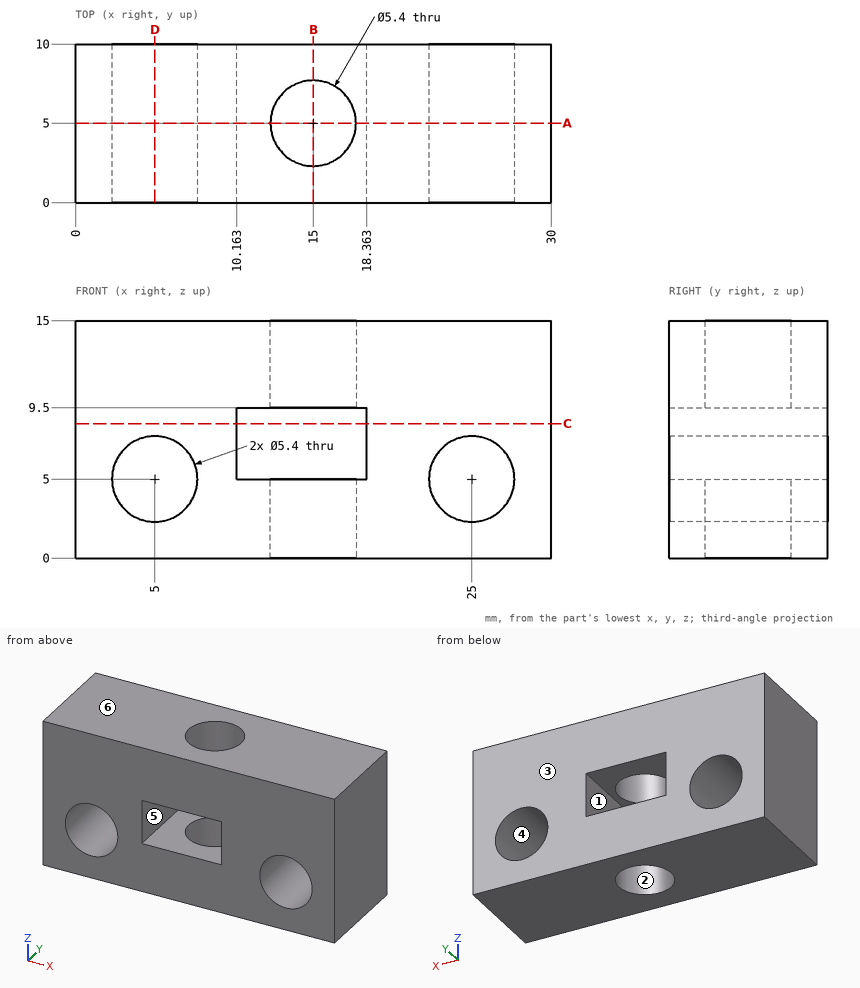
Geometry check sheet. Reference: drawing and pictorial views, mm from the part's lowest x, y, z. A direction names the side the tool comes from. Give positions to 0.01 mm unless a question says otherwise; leave off trailing zeros. Loops run counter-clockwise (first coordinate to the right, second up) from the corner with the lowest first, then second, coordinate; pieces in that order, holes last. Notation, with made-up numbers: M -15.5,29.25 L 3.5,29.25 A25 ccw 3.5,45.25 Z; hole C 24,84 d3. An arc over 180 degrees is marked long. One line per question, with ' | ' between items.
Item 1: Draft check along Z on the marked faces 3, 4, 5 and 6. Enter one of: +Z half, -Z half, draft (parallel to the pull), parting line (faces both ways), or undercut.
Completed:
face 3: draft | face 4: undercut | face 5: undercut | face 6: +Z half
Item 2: Section check A-A, the plane y = 5. Record the cut outline in (x, z).
Completed:
outline: M 0,0 L 12.3,0 L 12.3,5 L 10.16,5 L 10.16,9.5 L 12.3,9.5 L 12.3,15 L 0,15 Z; M 17.7,0 L 30,0 L 30,15 L 17.7,15 L 17.7,9.5 L 18.36,9.5 L 18.36,5 L 17.7,5 Z; hole C 5,5 d5.4; hole C 25,5 d5.4
Item 3: Section check D-D, the plane x = 5. Record the cut outline in (y, z), plus the area to 3 significant figures.
Completed:
outline: M 0,0 L 10,0 L 10,2.3 L 0,2.3 Z; M 0,7.7 L 10,7.7 L 10,15 L 0,15 Z | area: 96.0 mm^2
Item 4: Section check C-C, the plane z = 8.5. Record the cut outline in (x, y), plus the area to 3 significant figures.
Completed:
outline: M 0,0 L 10.16,0 L 10.16,10 L 0,10 Z; M 18.36,0 L 30,0 L 30,10 L 18.36,10 Z | area: 218 mm^2
Item 5: Section check B-B, the plane x = 15. Record the cut outline in (y, z), plus the area to 3 significant figures.
Completed:
outline: M 0,0 L 2.3,0 L 2.3,5 L 0,5 Z; M 0,9.5 L 2.3,9.5 L 2.3,15 L 0,15 Z; M 7.7,0 L 10,0 L 10,5 L 7.7,5 Z; M 7.7,9.5 L 10,9.5 L 10,15 L 7.7,15 Z | area: 48.3 mm^2
Item 6: Thickness scan on line 1 (Y direction, x = 15, z = 13.4); line 2 (Z direction, x = 12, y = 2.75); line 3 (X direction, y = 5.25, z = 4.5). Record the ranges inside material, lowest first. Write a range as [from, to].
Completed:
line 1: y = [0, 2.3], [7.7, 10] | line 2: z = [0, 5], [9.5, 15] | line 3: x = [0, 2.35], [7.65, 12.31], [17.69, 22.35], [27.65, 30]
Item 7: Tool access check on the marked faces 1 and 2. Record the directions out of +Z, -Z, +X, -X, +Y, -Y that give a thin tool (end or side, any length) a straight path to the whole face; none if there is none.
Completed:
face 1: +Y, -Y | face 2: +Z, -Z
